CAD build for the part. Positions are in the model's coordinates, mm. A direction names the side the tool comes from. Give positions to 0.01 mm unless a question says otherwise; leave off trailing zeros. Loops run counter-clockwise (first coordinate to the right, second up) from the corner with the lowest first, then second, coordinate; pieces in that order, holes last.
Item 1: Saw through at B-B on z = -14. Give the cut face in (x, y), plus the area to 3 significant figures.
Item 2: Saw through at C-C on y = -3.75. Give the cut face in (x, z), plus the area to 3 significant figures.
Item 3: Drop flat-ended pins along their axis: P1, Ø6, axis at x = 78, y = 3, coming from the -Z side; P2, Ø0.8, axis at y = 1, z = -40, coming from the +X side; P3, Ø5, axis at y = 6.5, z = -18, coming from the -X side; P4, Ø10, axis at x = 50.5, y = 8, coming from the +Z side. Give the stop position or say it passes through.
Item 4: Saw through at D-D on z = -42. Give the cut face in (x, y), plus the area to 3 significant figures.
Item 5: Which spindle directions (+Z, -Z, +X, -X, +Y, -Y) get a long thin tool onto all of the face, cutting with end or side? Do faces 4 (the flat face through (8, -5, -34.54)), 5 (the flat face through (61.618, 1, -41)), 6 (the flat face through (11.27, 1, -19)). Say none if no direction does.
Item 6: Mould opens along X. For faces 1 (the flat face through (76, 1, -33)), 2 (the flat face through (24, 1, -24.352)), 3 (the flat face through (59.078, 8, -16)) say: released by +X, released by -X, zero draft, split by the parting line, or undercut.
Item 7: Saw through at A-A on x = 40. Give the cut face in (y, z).
Item 8: Probe probe 1 along X at (y, z) = (1.55, -42); probe 2 along X at (y, z) = (2.75, -18.5); probe 3 along X at (y, z) = (1.7, -4). List the from-to ranges inside material, lowest first.
from build123d import *

# Parameters (mm, degrees)
SKETCH1_W           = 61.618
SKETCH1_H           = 50
SKETCH1_R           = 3.5
SKETCH1_R_2         = 1
SKETCH1_W_2         = 30.0482
SKETCH1_H_2         = 11.43
BOSS_EXTRUDE1_DEPTH = 2.54
BOSS_EXTRUDE2_DEPTH = 10.16
BOSS_EXTRUDE3_START = -32
BOSS_EXTRUDE3_DEPTH = 32
SKETCH5_W           = 29.558
SKETCH5_H           = 10
BOSS_EXTRUDE4_DEPTH = 2
SKETCH9_W           = 8.561459742
SKETCH9_H           = 33.54
CUT_EXTRUDE1_DEPTH  = 10.16
SKETCH10_R          = 1.65
SKETCH10_R_2        = 1.5
CUT_EXTRUDE2_DEPTH  = 107.976533202
BOSS_EXTRUDE7_DEPTH = 10
SKETCH12_R          = 4
BOSS_EXTRUDE8_DEPTH = 1
SKETCH13_W          = 12
SKETCH13_H          = 10
CUT_EXTRUDE3_DEPTH  = 10
SKETCH14_W          = 3.302
SKETCH14_H          = 11.43
BOSS_EXTRUDE9_DEPTH = 2.54


with BuildPart() as part:
    # Sketch1 → Boss-Extrude1 (new body)
    with BuildSketch(Plane(origin=(0, 0, 0), x_dir=(1, 0, 0), z_dir=(0, 1, 0))):
        with Locations((30.809, 25)):
            Rectangle(SKETCH1_W, SKETCH1_H)
        with Locations(Location((15, 42, 0), (0, 0, 270))):
            Circle(SKETCH1_R, mode=Mode.SUBTRACT)
        with Locations(Location((40, 42, 0), (0, 0, 270))):
            Circle(SKETCH1_R, mode=Mode.SUBTRACT)
        with Locations(Location((12.524, 4.6002, 0), (0, 0, 270))):
            Circle(SKETCH1_R_2, mode=Mode.SUBTRACT)
        with Locations((26.2941, 18.637)):
            Rectangle(SKETCH1_W_2, SKETCH1_H_2, mode=Mode.SUBTRACT)
    extrude(amount=BOSS_EXTRUDE1_DEPTH)

    # Sketch3 → Boss-Extrude2 (add)
    with BuildSketch(Plane.XZ):
        Polygon((10, -32), (10, -2), (15, -2), (15, 0), (7.46, 0), (7.46, -34.54), (10, -34.54), align=None)
    extrude(amount=BOSS_EXTRUDE2_DEPTH)

    # Sketch4 → Boss-Extrude3 (add)
    with BuildSketch(Plane.XY.offset(BOSS_EXTRUDE3_START)):
        Polygon((59.078, 0), (59.078, 12.54), (93.716, 12.54), (93.716, 0), (91.176, 0), (91.176, 10), (61.618, 10), (61.618, 0), align=None)
    extrude(amount=BOSS_EXTRUDE3_DEPTH)

    # Sketch5 → Boss-Extrude4 (add)
    with BuildSketch(Plane.XY):
        with Locations((76.397, 5)):
            Rectangle(SKETCH5_W, SKETCH5_H)
    extrude(amount=-BOSS_EXTRUDE4_DEPTH)

    # Sketch9 → Cut-Extrude1 (cut)
    with BuildSketch(Plane.XZ.offset(10.16)):
        with Locations((13.780729871, -18.27)):
            Rectangle(SKETCH9_W, SKETCH9_H)
    extrude(amount=-CUT_EXTRUDE1_DEPTH, mode=Mode.SUBTRACT)

    # Sketch10 → Cut-Extrude2 (cut, through all)
    with BuildSketch(Plane(origin=(0, 2.54, 0), x_dir=(1, 0, 0), z_dir=(0, 1, 0))):
        with Locations(Location((57.618, 46, 0), (0, 0, 270))):
            Circle(SKETCH10_R)
        with Locations(Location((4, 4, 0), (0, 0, 270))):
            Circle(SKETCH10_R)
        with Locations(Location((12.524, 4.6002, 0), (0, 0, 270))):
            Circle(SKETCH10_R_2)
    extrude(amount=-CUT_EXTRUDE2_DEPTH, mode=Mode.SUBTRACT)

    # Sketch11 → Boss-Extrude7 (add)
    with BuildSketch(Plane.XZ):
        Polygon((91.176, -32), (93.716, -32), (93.716, 0), (61.618, 0), (61.618, -2), (91.176, -2), align=None)
    extrude(amount=BOSS_EXTRUDE7_DEPTH)

    # Sketch12 → Boss-Extrude8 (add)
    with BuildSketch(Plane(origin=(0, 0, -32), x_dir=(-1, 0, 0), z_dir=(0, 0, -1))):
        Polygon((-59.078, 2.54), (-61.618, 2.54), (-61.618, -10), (-93.716, -10), (-93.716, 12.54), (-59.078, 12.54), align=None)
        with Locations((-85.4356, 4.031)):
            Circle(SKETCH12_R, mode=Mode.SUBTRACT)
    extrude(amount=BOSS_EXTRUDE8_DEPTH)

    # Sketch13 → Cut-Extrude3 (cut)
    with BuildSketch(Plane.XY):
        with Locations((67.618, -5)):
            Rectangle(SKETCH13_W, SKETCH13_H)
    extrude(amount=-CUT_EXTRUDE3_DEPTH, mode=Mode.SUBTRACT)

    # Sketch14 → Boss-Extrude9 (add)
    with BuildSketch(Plane(origin=(0, 2.54, 0), x_dir=(1, 0, 0), z_dir=(0, 1, 0))):
        with Locations((39.6672, 18.637)):
            Rectangle(SKETCH14_W, SKETCH14_H)
    extrude(amount=-BOSS_EXTRUDE9_DEPTH)


solid = part.part
Results below:
1. outline: (0, 0) - (7.46, 0) - (7.46, -10.16) - (9.5, -10.16) - (9.5, 0) - (11.27, 0) - (11.27, 2.54) - (0, 2.54) - close; (38.02, 0) - (61.62, 0) - (61.62, 10) - (91.18, 10) - (91.18, -10) - (93.72, -10) - (93.72, 12.54) - (59.08, 12.54) - (59.08, 2.54) - (38.02, 2.54) - close
1. area: 267 mm2
2. outline: (7.46, -34.54) - (9.5, -34.54) - (9.5, -1.5) - (15, -1.5) - (15, 0) - (7.46, 0) - close; (61.62, -33) - (93.72, -33) - (93.72, 0) - (73.62, 0) - (73.62, -2) - (91.18, -2) - (91.18, -32) - (61.62, -32) - close
2. area: 227 mm2
3. P1: stops at z = -33
3. P2: stops at x = 61.62
3. P3: stops at x = 59.08
3. P4: passes through
4. outline: (0, 0) - (11.5, 0) - (11.5, 2.54) - (0, 2.54) - close; (18.5, 0) - (36.5, 0) - (36.5, 2.54) - (18.5, 2.54) - close; (43.5, 0) - (61.62, 0) - (61.62, 2.54) - (43.5, 2.54) - close
4. area: 121 mm2
5. face 4: -Z, +X, -X, -Y
5. face 5: -Z, +X, +Y, -Y
5. face 6: +Y, -Y
6. face 1: zero draft
6. face 2: undercut
6. face 3: released by -X
7. outline: (0, -50) - (2.54, -50) - (2.54, -45.5) - (0, -45.5) - close; (0, -38.5) - (2.54, -38.5) - (2.54, 0) - (0, 0) - close
8. probe 1: x = 0 to 11.5, 18.5 to 36.5, 43.5 to 61.62
8. probe 2: x = 59.08 to 61.62, 91.18 to 93.72
8. probe 3: x = 0 to 2.35, 5.65 to 11.15, 13.9 to 61.62, 91.18 to 93.72
